Geometry: final body of the model. Coordinates: model frame, mm. Coordinates: 2 decimals unless noted, no trailing zeros. Write each loop counter-clockwise with the first axis right and the second up, starting at its lowest first coordinate (ties: lowest second). Pieces come first, ordered by that corner, then holes. Notation, with made-up numbers: (82, 83) - (87, 83) arc R6 cw to (87, 93) - close; hole circle Ø10 at (-9, 38). An arc over 180 degrees is marked (long way). Answer as a JSON object with one key per item and string values. Group by question number.
Item 1: Section A-A on z = -14. Return loops of the section in (x, y).
Item 2: First-contact query: pin 1 Ø0.8 at (y, z) = (-1, 37.5) entering from -X; pin 2 Ø0.5 at (y, z) = (-0.5, -36.5) entering from +X; pin 3 Ø0.8 at (y, z) = (-0.5, 15) entering from +X. Flat tips, straight axial feed; report the tip coordinate or a pass-through.
Item 3: Section B-B on x = -2. Return loops of the section in (y, z), and give its area (3 significant figures).
Item 4: Line query: line 1 along Z through (x, y) = (15, -0.3); line 2 along X through (y, z) = (-0.45, 17.5); line 3 along X through (y, z) = (-0.25, 29). Output: solid intervals per line, ascending. Write a range as from..to.
```python
from build123d import *

# Parameters (mm, degrees)
F0_W     = 6.35
F0_H     = 2.032
F0_W_2   = 72.136
F0_H_2   = 24.384
F0_W_3   = 1.651
F1_DEPTH = 1.524


with BuildPart() as f1:
    # F0 (on Front) → F1 (new body)
    with BuildSketch(Plane.XZ):
        with BuildLine():
            Line((18.418700083, 36.344532257), (9.1906381628, 36.344532257))
            Line((9.1906381628, 36.344532257), (2.8406381628, 36.344532257))
            Line((2.8406381628, 36.344532257), (-8.5829475322, 36.344532257))
            Line((-8.5829475322, 36.344532257), (-14.9329475322, 36.344532257))
            Line((-14.9329475322, 36.344532257), (-24.1610094524, 36.344532257))
            ThreePointArc((-24.1610094524, 36.344532257), (-26.5910492479, 35.8611672884), (-28.6511375129, 34.4846603175))
            Line((-28.6511375129, 34.4846603175), (-37.0792827452, 26.0565150852))
            ThreePointArc((-37.0792827452, 26.0565150852), (-38.4557897162, 23.9964268202), (-38.9391546847, 21.5663870246))
            Line((-38.9391546847, 21.5663870246), (-38.9391546847, 12.468532257))
            Line((-38.9391546847, 12.468532257), (33.1968453153, 12.468532257))
            Line((33.1968453153, 12.468532257), (33.1968453153, 21.5663870246))
            ThreePointArc((33.1968453153, 21.5663870246), (32.7134803467, 23.9964268202), (31.3369733758, 26.0565150852))
            Line((31.3369733758, 26.0565150852), (22.9088281435, 34.4846603175))
            ThreePointArc((22.9088281435, 34.4846603175), (20.8487398785, 35.8611672884), (18.418700083, 36.344532257))
        make_face()
        with Locations((-11.7579475322, 37.360532257)):
            Rectangle(F0_W, F0_H)
        with Locations((6.0156381628, 37.360532257)):
            Rectangle(F0_W, F0_H)
        with Locations((-11.7579475322, -36.807467743)):
            Rectangle(F0_W, F0_H)
        with Locations((6.0156381628, -36.807467743)):
            Rectangle(F0_W, F0_H)
        with BuildLine():
            Line((33.1968453153, -21.0133225107), (33.1968453153, -11.915467743))
            Line((33.1968453153, -11.915467743), (-38.9391546847, -11.915467743))
            Line((-38.9391546847, -11.915467743), (-38.9391546847, -21.0133225107))
            ThreePointArc((-38.9391546847, -21.0133225107), (-38.4557897162, -23.4433623062), (-37.0792827452, -25.5034505712))
            Line((-37.0792827452, -25.5034505712), (-28.6511375129, -33.9315958036))
            ThreePointArc((-28.6511375129, -33.9315958036), (-26.5910492479, -35.3081027745), (-24.1610094524, -35.791467743))
            Line((-24.1610094524, -35.791467743), (-14.9329475322, -35.791467743))
            Line((-14.9329475322, -35.791467743), (-8.5829475322, -35.791467743))
            Line((-8.5829475322, -35.791467743), (2.8406381628, -35.791467743))
            Line((2.8406381628, -35.791467743), (9.1906381628, -35.791467743))
            Line((9.1906381628, -35.791467743), (18.418700083, -35.791467743))
            ThreePointArc((18.418700083, -35.791467743), (20.8487398785, -35.3081027745), (22.9088281435, -33.9315958036))
            Line((22.9088281435, -33.9315958036), (31.3369733758, -25.5034505712))
            ThreePointArc((31.3369733758, -25.5034505712), (32.7134803467, -23.4433623062), (33.1968453153, -21.0133225107))
        make_face()
        with Locations((-2.8711546847, 0.276532257)):
            Rectangle(F0_W_2, F0_H_2)
        with Locations((-39.7646546847, 0.276532257)):
            Rectangle(F0_W_3, F0_H_2)
        with Locations((34.0223453153, 0.276532257)):
            Rectangle(F0_W_3, F0_H_2)
    extrude(amount=F1_DEPTH)


solid = f1.part
```
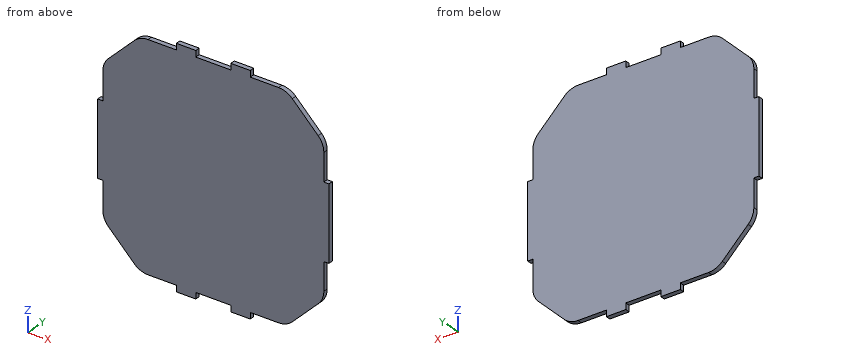
Checks:
{
 "1": {"outline": "(-38.94, -1.52) - (33.2, -1.52) - (33.2, 0) - (-38.94, 0) - close"},
 "2": {"pin 1": "x = -14.93", "pin 2": "x = 9.19", "pin 3": "x = 33.2"},
 "3": {"outline": "(-1.52, -35.79) - (0, -35.79) - (0, 36.34) - (-1.52, 36.34) - close", "area": "110 mm^2"},
 "4": {"line 1": "-35.79..36.34", "line 2": "-38.94..33.2", "line 3": "-34.14..28.39"}
}
